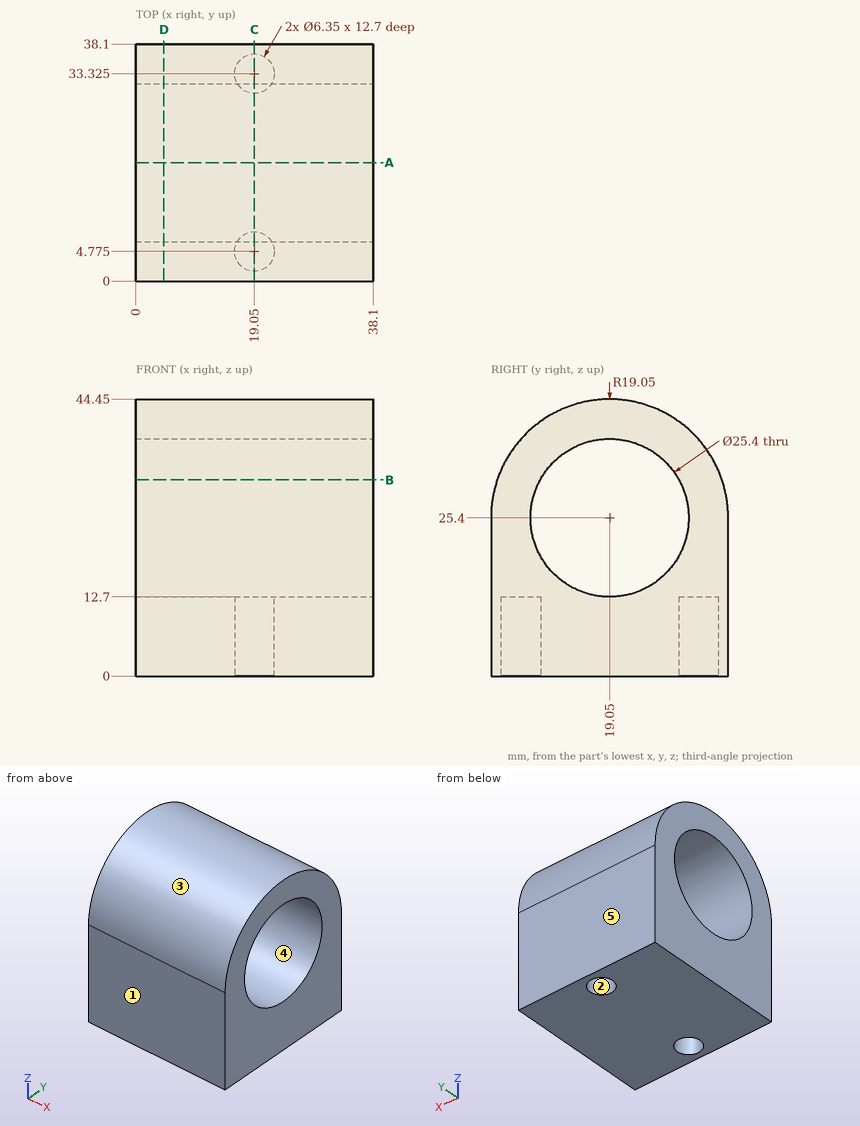
Print and shaded views of the part. All mm, measured from the part's lowest x, y and z. A direction names the side the tool comes from. Coordinates: 2 decimals unless noted, no trailing zeros. Loops run counter-clockwise (first coordinate to the right, second up) from the corner with the lowest first, then second, coordinate; pieces in that order, holes last. Notation, with made-up numbers: M 29,11.5 L 67,11.5 A13 ccw 67,18.5 Z; hole C -19,-12.75 d9. An arc over 180 degrees is marked long. Use a Markdown table: item, result. Add a question column.
Q1. Cut at D-D (x = 4.5). Write the cut outline in (y, z).
Q2. Cut at C-C (x = 19.05). Write the cut outline in (y, z), and give its area (3 significant figures).
Q3. Pin check, flat tips, straight feed: P1, Ø5, axis at y = 14.5, z = 14.5, coming from the -X side; P2, Ø4, axis at x = 19.05, y = 4.78, coming from the +Z side; P3, Ø5, axis at x = 16.5, y = 12, coming from the +Z side; P4, Ø1, axis at x = 7.5, y = 13.5, coming from the +Z side. Stop position of each tip, or through.
Q4. Probe L1, parallel to Y at x = 19, z = 3; L2, parallel to Z at x = 2.5, y = 19.5 (1 decimal); L3, parallel to Y at x = 28, z = 25. List the from-to ranges inside material, lowest first.
Q5. Mould opens along Z. For the marked faces 3, 4 and 5 say: +Z half, -Z half, draft (parallel to the pull), parting line (faces both ways), or undercut.
Q6. Cut at A-A (y = 19.05). Write the cut outline in (x, z).
Q7. Which spindle directions (+Z, -Z, +X, -X, +Y, -Y) get a long thin tool onto all of the face, cutting with end or side? Do the marked faces 1 and 2. Say none if no direction does.
Q8. Cut at B-B (z = 31.5). Write the cut outline in (x, y).
Worked out:
| question | item | result |
|---|---|---|
| 1 | outline | M 0,0 L 38.1,0 L 38.1,25.4 A19.05 ccw 0,25.4 Z; hole C 19.05,25.4 d25.4 |
| 2 | outline | M 0,0 L 1.6,0 L 1.6,12.7 L 7.95,12.7 L 7.95,0 L 30.15,0 L 30.15,12.7 L 36.5,12.7 L 36.5,0 L 38.1,0 L 38.1,25.4 A19.05 ccw 0,25.4 Z; hole C 19.05,25.4 d25.4 |
| 2 | area | 870 mm2 |
| 3 | P1 | stops at x = 0 |
| 3 | P2 | stops at z = 39.97 |
| 3 | P3 | stops at z = 43.9 |
| 3 | P4 | stops at z = 43.77 |
| 4 | L1 | y = 0 to 1.6, 7.95 to 30.15, 36.5 to 38.1 |
| 4 | L2 | z = 0 to 12.7, 38.1 to 44.4 |
| 4 | L3 | y = 0 to 6.36, 31.74 to 38.1 |
| 5 | face 3 | +Z half |
| 5 | face 4 | undercut |
| 5 | face 5 | draft |
| 6 | outline | M 0,0 L 38.1,0 L 38.1,12.7 L 0,12.7 Z; M 0,38.1 L 38.1,38.1 L 38.1,44.45 L 0,44.45 Z |
| 7 | face 1 | +Z, -Z, +X, -X, -Y |
| 7 | face 2 | -Z |
| 8 | outline | M 0,1 L 38.1,1 L 38.1,7.91 L 0,7.91 Z; M 0,30.19 L 38.1,30.19 L 38.1,37.1 L 0,37.1 Z |
